Solid Edge part; units mm, degrees
sketch "Sketch1" plane through (0, 0, 0) normal (0, 0, 1) x (1, 0, 0)
  line L0 (-220, -220) -> (220, -220)
  line L1 (220, -220) -> (220, 220)
  line L2 (220, 220) -> (-220, 220)
  line L3 (-220, 220) -> (-220, -220)
extrude "Protrusion1" add sketch "Sketch1" along normal blind 20
fillet "Round_1" radius 1.5 12 edges at (0, 220, 20) (220, 0, 20) (0, -220, 20) (-220, 0, 20) (-220, -220, 10) (220, -220, 10) (-220, 220, 10) (220, 220, 10) (0, 220, 0) (-220, 0, 0) (220, 0, 0) (0, -220, 0)
hole "Hole_7" at (189.9692, -180, 0) direction (0, 0, 1) diameter 10 depth 15
hole "Hole1" at (190, 0, 0) direction (0, 0, 1) diameter 10 depth 15
hole "Hole2" at (190, 180, 0) direction (0, 0, 1) diameter 10 depth 15
mirror "Mirror1" about plane through (0, 0, 0) normal (1, 0, 0) of "Hole_7", "Hole1", "Hole2"
properties material "Wood, Oak"
Geometry: final body of the model. Coordinates: model frame, mm. A direction names the side the tool comes from. Give positions to 0.01 mm unless a question says otherwise; leave off trailing zeros. Loops run counter-clockwise (first coordinate to the right, second up) from the corner with the lowest first, then second, coordinate; pieces in that order, holes last. Notation, with made-up numbers: M -14,56.5 L 41,56.5 A18 ccw 41,62.5 Z; hole C -35.75,13.25 d7. An arc over 180 degrees is marked long. Put each result on its own line as item: value. Start each with the question number.
1) Ray query, line 1 along X through (y, z) = (-180, 9.5); line 2 along Y through (x, z) = (190, 3); line 3 along X through (y, z) = (-97, 19.25). Return the intervals inside material, ascending.
2) Pull-direction query (X, two-part tool) for faces 1 (the cylindrical face through (185.043, -0.651, 7.605)), 2 (the flat face through (-3, -220, 10)), 3 (the flat face through (-220, 3, 10)); classes: pulls with the +X half, pulls with the -X half, needs draft (parallel to the pull), parting line crosses it, or undercut.
3) Contact query for a flat-ended pin moving along its axis: pin 1 (3 mm diameter, centred on x = -190.5, y = 1, fed in from -Z). Output: stop coordinate, or through.
4) Access query for faces 4 (the flat face through (190, 180, 15)), 5 (the flat face through (-3, 3, 20)). Directions: +Z, -Z, +X, -X, +Y, -Y. A direction counts if a zero-diameter tool reaches every point of the face in a straight line with its end or side. Return the directions, or none.
5) Cut plane A-A (y = -180). Output: boundary loops of the cut face in (x, z).
Verdict:
1. line 1: -220 to -194.97, -184.97 to 184.97, 194.97 to 220
1. line 2: -220 to -185, -175 to -5, 5 to 175, 185 to 220
1. line 3: -219.8 to 219.8
2. face 1: undercut
2. face 2: needs draft
2. face 3: pulls with the -X half
3. pin 1: z = 15
4. face 4: -Z
4. face 5: +Z, +X, -X, +Y, -Y
5. outline: M -220,1.5 A1.5 ccw -218.5,0 L -194.97,0 L -194.97,15 L -184.97,15 L -184.97,0 L 184.97,0 L 184.97,15 L 194.97,15 L 194.97,0 L 218.5,0 A1.5 ccw 220,1.5 L 220,18.5 A1.5 ccw 218.5,20 L -218.5,20 A1.5 ccw -220,18.5 Z
